from build123d import *

# Parameters (mm, degrees)
SKETCH1_R                = 30
BOSS_EXTRUDE1_DEPTH      = 25
CHAMFER1_SIZE            = 6
BOSS_EXTRUDE2_REACH      = 149.272
BOSS_EXTRUDE2_END_RADIUS = 30
SKETCH2_R                = 15
SKETCH3_R                = 22.5
BOSS_EXTRUDE3_DEPTH      = 24
CHAMFER2_SIZE            = 2
SKETCH4_R                = 15
CUT_EXTRUDE1_DEPTH       = 10


with BuildPart() as part:
    # Sketch1 → Boss-Extrude1 (new, symmetric)
    with BuildSketch(Plane.XY):
        Circle(SKETCH1_R)
    extrude(amount=BOSS_EXTRUDE1_DEPTH, both=True)

    # Chamfer1
    chamfer1_edges = [part.edges().sort_by_distance(p)[0] for p in [
        (-30, 0, 25),
    ]]
    chamfer(chamfer1_edges, length=CHAMFER1_SIZE)

    # Boss-Extrude2: up to this cylinder (the profile starts outside it)
    boss_extrude2_end = Plane(origin=(0, 0, 0), z_dir=(0, 0, -1)) * Cylinder(BOSS_EXTRUDE2_END_RADIUS, 359.544, mode=Mode.PRIVATE)
    # Sketch2 → Boss-Extrude2 (add, up to the surface)
    with BuildSketch(Plane(origin=(112, 0, 0), x_dir=(0, 0, -1), z_dir=(1, 0, 0)), mode=Mode.PRIVATE) as boss_extrude2_sk1:
        Circle(SKETCH2_R)
    boss_extrude2_tool1 = extrude(boss_extrude2_sk1.sketch, amount=-BOSS_EXTRUDE2_REACH, mode=Mode.PRIVATE) - boss_extrude2_end
    add(boss_extrude2_tool1.solids().sort_by_distance((112, 0, 0))[0])

    # Sketch3 → Boss-Extrude3 (add)
    with BuildSketch(Plane(origin=(72, 0, 0), x_dir=(0, 0, -1), z_dir=(1, 0, 0))):
        Circle(SKETCH3_R)
    extrude(amount=-BOSS_EXTRUDE3_DEPTH)

    # Chamfer2
    chamfer2_edges = [part.edges().sort_by_distance(p)[0] for p in [
        (48, 0, 22.5),
        (72, 0, 22.5),
    ]]
    chamfer(chamfer2_edges, length=CHAMFER2_SIZE)

    # Sketch4 → Cut-Extrude1 (cut)
    with BuildSketch(Plane(origin=(0, 0, -25), x_dir=(-1, 0, 0), z_dir=(0, 0, -1))):
        Circle(SKETCH4_R)
    extrude(amount=-CUT_EXTRUDE1_DEPTH, mode=Mode.SUBTRACT)


solid = part.part
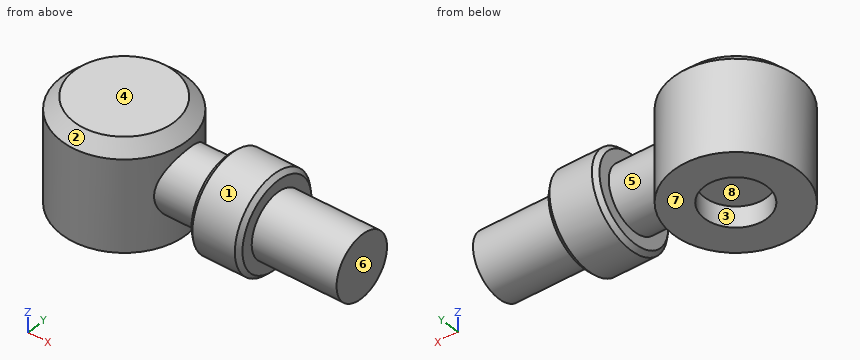
The listing builds one solid part. Answer for the finished solid, in the listing's coordinates (mm). Face numbers are marked on the shaded views. A direction names the side the tool comes from. Round coordinates to 2 decimals unless told otherwise and drop trailing zeros. Order: outer loops, then holes, each group sorted by start corner. A loop starts at its lowest first (then second) coordinate and runs counter-clockwise, first axis right, second up. Notation, with made-up numbers: (13, 74) -> (65, 74) arc R8 cw to (65, 80) -> close; hole circle Ø9 at (16, 16). An arc over 180 degrees is marked (long way). Put each result on its own line as item: value.
Q1. Section A-A, the plane z = 0 is taken. Write down the section's boundary in (x, y), and give its area (3 significant figures).
Results list:
outline: (25.98, -15) -> (48, -15) -> (48, -20.5) -> (50, -22.5) -> (70, -22.5) -> (72, -20.5) -> (72, -15) -> (112, -15) -> (112, 15) -> (72, 15) -> (72, 20.5) -> (70, 22.5) -> (50, 22.5) -> (48, 20.5) -> (48, 15) -> (25.98, 15) arc R30 ccw (long way) to start
area: 5,680 mm^2
Q2. Each of these flat-tipped pins is pushed along its axis until it touches: P1, Ø12, axis at x = 10.5, z = 16.5, coming from the -Y side; P2, Ø6, axis at x = 49.5, z = 13.5, coming from the +Y side; P3, Ø4, axis at x = 81, y = -6, coming from the -Z side. Where does it stop, or does it pass through?
Results list:
P1: y = -29.66
P2: y = 19.88
P3: z = -14.46
Q3. Section B-B, the plane y = 0 is taken. Write down the section's boundary in (x, z), and give its area (3 significant figures).
Results list:
outline: (-30, -25) -> (-15, -25) -> (-15, -15) -> (15, -15) -> (15, -25) -> (30, -25) -> (30, -15) -> (48, -15) -> (48, -20.5) -> (50, -22.5) -> (70, -22.5) -> (72, -20.5) -> (72, -15) -> (112, -15) -> (112, 15) -> (72, 15) -> (72, 20.5) -> (70, 22.5) -> (50, 22.5) -> (48, 20.5) -> (48, 15) -> (30, 15) -> (30, 19) -> (24, 25) -> (-24, 25) -> (-30, 19) -> close
area: 5,480 mm^2
Q4. Section C-C, the plane x = 0 is taken. Write down the section's boundary in (y, z), and give its area (3 significant figures).
Results list:
outline: (-30, -25) -> (-15, -25) -> (-15, -15) -> (15, -15) -> (15, -25) -> (30, -25) -> (30, 19) -> (24, 25) -> (-24, 25) -> (-30, 19) -> close
area: 2,660 mm^2
Q5. Determine the mould class of the marked faces 6, 7 and 8 for opening direction X: pulls with the +X half, pulls with the -X half, needs draft (parallel to the pull), parting line crosses it, or undercut.
Results list:
face 6: pulls with the +X half
face 7: needs draft
face 8: undercut
Q6. Section D-D, the plane x = 40 is taken. Write down the section's boundary in (y, z).
Results list:
outline: circle Ø30 at (0, 0)
Q7. Consider line 1 along Y through (x, z) = (0, -17.25); line 2 along X through (y, z) = (2, 20); line 3 along X through (y, z) = (-1, 4.5). Determine where each line is inside the solid, lowest interval first.
Results list:
line 1: -30 to -15, 15 to 30
line 2: -28.93 to 28.93, 48 to 72
line 3: -29.98 to 112
Q8. Which of the six approach directions +Z, -Z, +X, -X, +Y, -Y give full straight-line access (tool end or side, diameter ignored) to the marked faces 1, 2, 3, 4 and 5?
Results list:
face 1: +X
face 2: +Z
face 3: -Z
face 4: +Z, +X, -X, +Y, -Y
face 5: none
